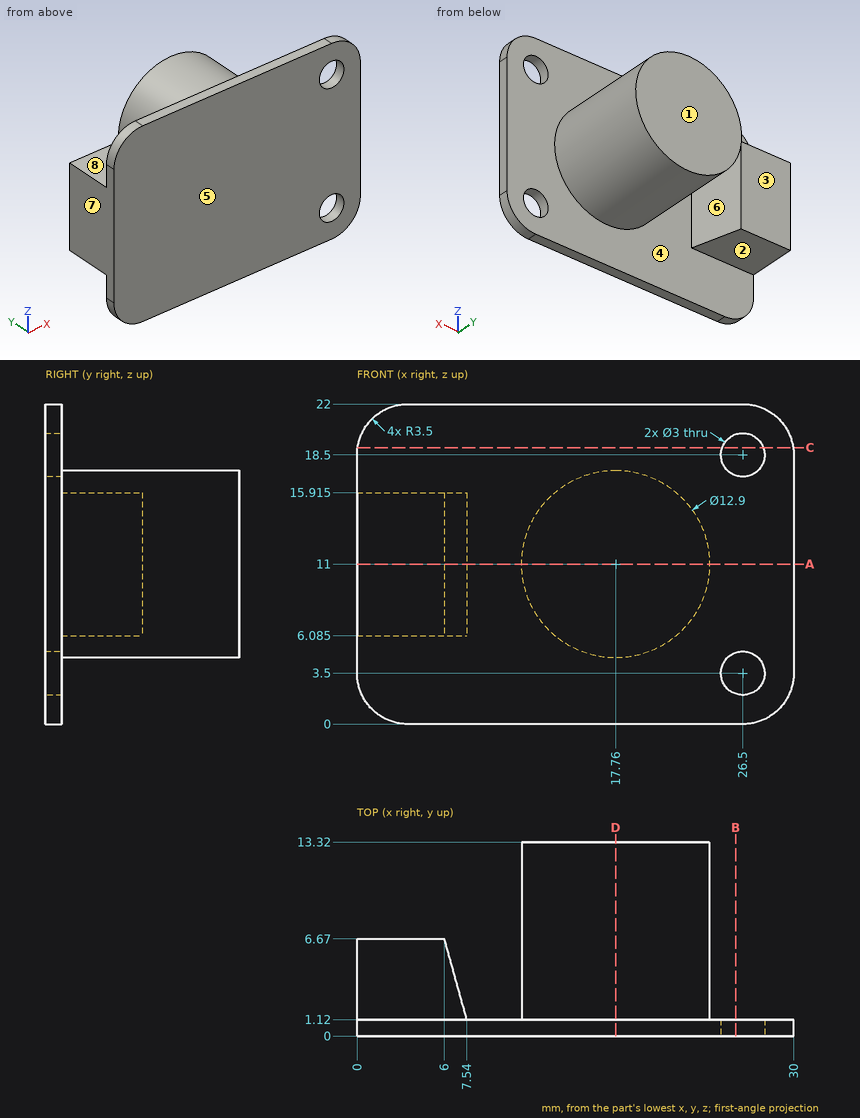
Geometry check sheet. Reference: drawing and pictorial views, mm from the part's lowest x, y, z. A direction names the side the tool comes from. Round coordinates to 2 decimals unless told otherwise and drop trailing zeros. Order: outer loops, then holes, each group sorted by start corner. A loop starts at its lowest first (then second) coordinate and runs counter-clockwise, first axis right, second up.
Q1. Cross-section at A-A, the plane z = 11. Enter the section's corners in (x, y).
Filled sheet:
outline: (0, 0) - (30, 0) - (30, 1.12) - (24.21, 1.12) - (24.21, 13.32) - (11.31, 13.32) - (11.31, 1.12) - (7.54, 1.12) - (6, 6.67) - (0, 6.67) - close
Q2. Draft check along X on the marked faces 6, 7 and 8. Enter one of: pulls with the +X half, pulls with the -X half, needs draft (parallel to the pull), parting line crosses it, or undercut.
Filled sheet:
face 6: undercut
face 7: pulls with the -X half
face 8: needs draft
Q3. Set-up check for the marked faces 1, 2, 3, 4 and 5: record each of +Z, -Z, +X, -X, +Y, -Y from which the full face is reachable in a straight line by a thin tool's end or side.
Filled sheet:
face 1: +Z, -Z, +X, -X, +Y
face 2: -Z, -X, +Y
face 3: +Z, -Z, -X, +Y
face 4: +Y
face 5: +Z, -Z, +X, -X, -Y
Q4. Depth check by flat-ended pin: P1, Ø2, axis at y = 10.5, z = 17.5, coming from the +X side; P2, Ø1.5, axis at x = 6, y = 7, coming from the +Z side (3 decimals); P3, Ø5, axis at x = 18, y = 12, coming from the -Z side. Enter the tip coordinate at first touch or a pass-through.
Filled sheet:
P1: stops at x = 21.13
P2: stops at z = 15.915
P3: stops at z = 4.55
Q5. Cross-section at D-D, the plane x = 17.76. Enter the section's corners in (y, z), plus the area to 3 significant figures.
Filled sheet:
outline: (0, 0) - (1.12, 0) - (1.12, 4.55) - (13.32, 4.55) - (13.32, 17.45) - (1.12, 17.45) - (1.12, 22) - (0, 22) - close
area: 182 mm2
Q6. Scan lines: L1, parallel to X at y = 0.7, z = 18.5; L2, parallel to Z at x = 6.5, y = 1.5 (3 decimals); L3, parallel to Y at x = 6.5, z = 3. Record each from-to range of solid material in increasing order.
Filled sheet:
L1: x = 0 to 25, 28 to 30
L2: z = 6.085 to 15.915
L3: y = 0 to 1.12
Q7. Cross-section at B-B, the plane x = 26. Enter the section's corners in (y, z), plus the area to 3 significant figures.
Filled sheet:
outline: (0, 0) - (1.12, 0) - (1.12, 2.09) - (0, 2.09) - close; (0, 4.91) - (1.12, 4.91) - (1.12, 17.09) - (0, 17.09) - close; (0, 19.91) - (1.12, 19.91) - (1.12, 22) - (0, 22) - close
area: 18.3 mm2
Q8. Cross-section at C-C, the plane z = 19. Enter the section's corners in (x, y).
Filled sheet:
outline: (0.04, 0) - (25.09, 0) - (25.09, 1.12) - (0.04, 1.12) - close; (27.91, 0) - (29.96, 0) - (29.96, 1.12) - (27.91, 1.12) - close
